Can you work these out from the drawing? Everything is in mm from the part's minimum corner. Give positions to 0.01 mm unless a question says otherwise; leave off trailing zeros. Write each loop counter-clockwise with the first axis right and the second up, starting at its lowest first coordinate (ties: lowest second). Pieces come first, ordered by that corner, then holes. Notation, with made-up numbers: (88.5, -18.75) - (96.5, -18.75) arc R20 cw to (96.5, 8.25) - close; hole circle Ø9 at (-18, 17). An arc over 180 degrees is marked (long way). Write each question's results on one line, items separated by ' | '. Start each with the question number.
Item 1: Suppose I cut it at A-A on x = 26.2. List the corners of the cut face in (y, z) for me, then the cut area to 3 significant figures.
Item 2: Suppose I cut it at B-B on z = 32.8. List the corners of the cut face in (x, y) for me, then the cut area to 3 significant figures.
Item 3: Please list where these lines run through material, in increasing order: line 1 along Z through (x, y) = (58, 1.8); line 2 along X through (y, z) = (0.8, 51.8); line 3 along X through (y, z) = (1.5, 51.2).
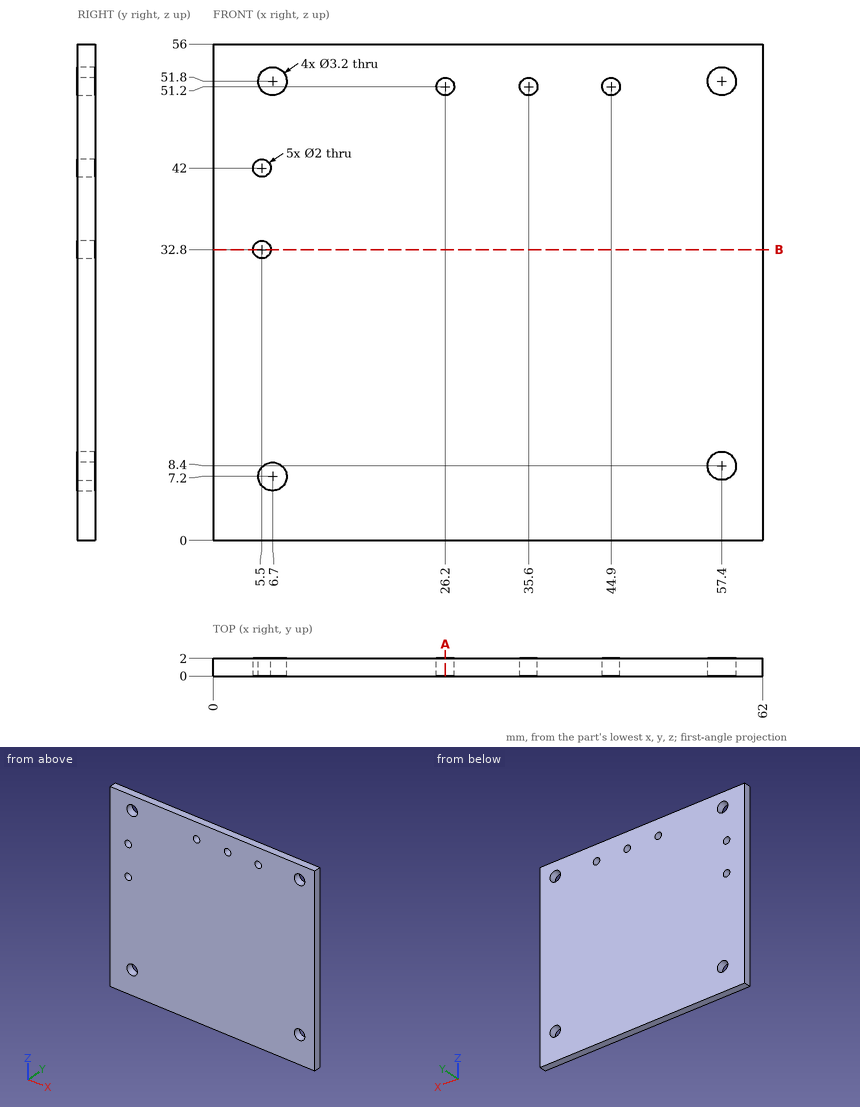
Checked values:
1) outline: (0, 0) - (2, 0) - (2, 50.2) - (0, 50.2) - close; (0, 52.2) - (2, 52.2) - (2, 56) - (0, 56) - close | area: 108 mm^2
2) outline: (0, 0) - (4.5, 0) - (4.5, 2) - (0, 2) - close; (6.5, 0) - (62, 0) - (62, 2) - (6.5, 2) - close | area: 120 mm^2
3) line 1: z = 0 to 6.92, 9.88 to 50.32, 53.28 to 56 | line 2: x = 0 to 5.1, 8.3 to 25.4, 27 to 34.8, 36.4 to 44.1, 45.7 to 55.8, 59 to 62 | line 3: x = 0 to 5.22, 8.18 to 25.2, 27.2 to 34.6, 36.6 to 43.9, 45.9 to 55.92, 58.88 to 62
